Can you work these out from the drawing? Everything is in mm from the part's minimum corner. A direction names the side the tool comes from. Give positions to 0.01 mm unless a question says otherwise; leave off trailing zeros. Loops run counter-clockwise (first coordinate to the right, second up) from the corner with the lowest first, then second, coordinate; pieces in that order, holes last. Notation, with made-up numbers: (43, 55.25) -> (97, 55.25) arc R23 cw to (97, 63.25) -> close; hole circle Ø4 at (45.25, 50.25). An arc over 180 degrees is marked (long way). Return JSON: item names as keys, results as strings. Group by question number.
Q1. Suppose I cut it at A-A, the plane x = 25. Please give me the cut outline in (y, z).
Q2. Suppose I cut it at B-B, the plane z = 13.7. Please give me the cut outline in (x, y), and give its area (3 significant figures).
Q3. Suppose I cut it at D-D, the plane x = 12. Please give me the cut outline in (y, z), and give its area (3 significant figures).
Q4. Thinking about a two-plate mould opening in Z: for the marked faces 4, 5 and 6, which applies, pulls with the +Z half, pulls with the -Z half, needs draft (parallel to the pull), parting line crosses it, or undercut?
Q5. Suppose I cut it at C-C, the plane y = 5. Please give me the cut outline in (x, z), and give its area (3 significant figures).
Q6. Which directions (+Z, -Z, +X, -X, +Y, -Y) give clear straight access to the entire face, cutting with the end or side of a thin tool? Please do the marked faces 1, 2 and 3.
Q7. Will these pins go through, and if not, where does the flat tip stop? pin 1 (7 mm diameter, centred on y = 16.5, z = 17, fed in from +X); pin 2 (5 mm diameter, centred on x = 22, z = 15, fed in from +Y).
Q8. I need wall thicknesses on line 1 along X through (y, z) = (23, 22); line 2 along X through (y, z) = (5.25, 29) (1 decimal). Which ranges of each line are inside material? Lowest first, please. Write a range as [from, to].
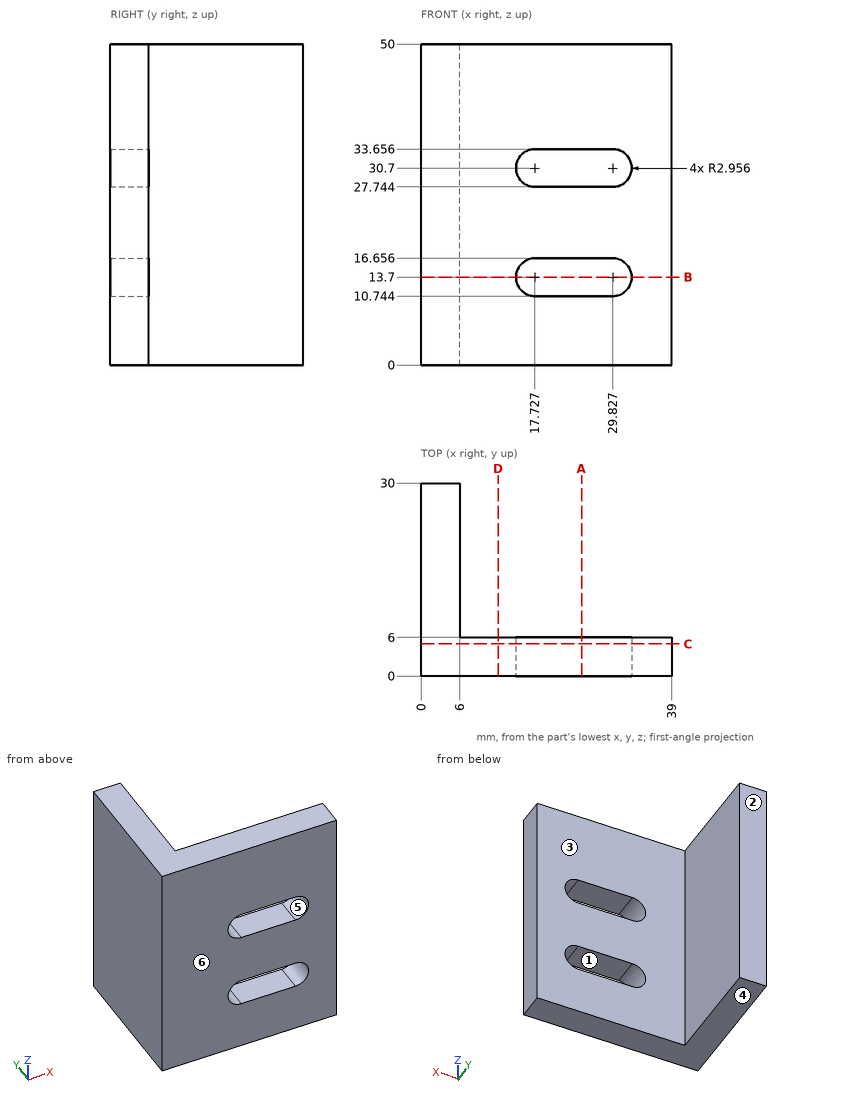
Ans:
{
 "1": {"outline": "(0, 0) -> (6, 0) -> (6, 10.74) -> (0, 10.74) -> close; (0, 16.66) -> (6, 16.66) -> (6, 27.74) -> (0, 27.74) -> close; (0, 33.66) -> (6, 33.66) -> (6, 50) -> (0, 50) -> close"},
 "2": {"outline": "(0, 0) -> (14.77, 0) -> (14.77, 6) -> (6, 6) -> (6, 30) -> (0, 30) -> close; (32.78, 0) -> (39, 0) -> (39, 6) -> (32.78, 6) -> close", "area": "270 mm^2"},
 "3": {"outline": "(0, 0) -> (6, 0) -> (6, 50) -> (0, 50) -> close", "area": "300 mm^2"},
 "4": {"face 4": "pulls with the -Z half", "face 5": "undercut", "face 6": "needs draft"},
 "5": {"outline": "(0, 0) -> (39, 0) -> (39, 50) -> (0, 50) -> close; hole (17.73, 10.74) -> (29.83, 10.74) arc R2.96 ccw to (29.83, 16.66) -> (17.73, 16.66) arc R2.96 ccw to start; hole (17.73, 27.74) -> (29.83, 27.74) arc R2.96 ccw to (29.83, 33.66) -> (17.73, 33.66) arc R2.96 ccw to start", "area": "1,750 mm^2"},
 "6": {"face 1": "+Y, -Y", "face 2": "+Z, -Z, +X, -X, +Y", "face 3": "+Z, -Z, +X, +Y"},
 "7": {"pin 1": "stops at x = 6", "pin 2": "stops at y = 6"},
 "8": {"line 1": "x = [0, 6]", "line 2": "x = [0, 15.3], [32.2, 39]"}
}
